Geometry: final body of the model. Coordinates: model frame, mm. A direction names the side the tool comes from. Coordinates: 2 decimals unless noted, no trailing zeros. Write each loop counter-clockwise with the first axis right and the second up, starting at its lowest first coordinate (ties: lowest second). Pieces come first, ordered by that corner, then holes. Notation, with made-up numbers: (6.5, 47) -> (23.5, 47) arc R17 ccw to (23.5, 78) -> close; hole circle Ø5 at (20, 77.25). An arc over 180 degrees is marked (long way). One line per item, written item: value.
```python
from build123d import *

# Parameters (mm, degrees)
SKETCH_1_R          = 27.5
EXTRUDE_1_DEPTH     = 4
SKETCH_2_R          = 25.4
EXTRUDE_2_DEPTH     = 3.175
SKETCH_3_R          = 1.6
CUT_EXTRUDE_1_DEPTH = 40.547194907
SKETCH_4_R          = 36
SKETCH_4_R_2        = 1.6
EXTRUDE_3_DEPTH     = 2


with BuildPart() as part:
    # ｽｹｯﾁ1 → ﾎﾞｽ - 押し出し1 (new body)
    with BuildSketch(Plane.XY):
        Circle(SKETCH_1_R)
    extrude(amount=EXTRUDE_1_DEPTH)

    # ｽｹｯﾁ2 → ﾎﾞｽ - 押し出し2 (add)
    with BuildSketch(Plane(origin=(0, 0, 0), x_dir=(-1, 0, 0), z_dir=(0, 0, -1))):
        Circle(SKETCH_2_R)
    extrude(amount=EXTRUDE_2_DEPTH)

    # ｽｹｯﾁ3 → ｶｯﾄ - 押し出し1 (cut, through all)
    with BuildSketch(Plane(origin=(0, 0, -3.175), x_dir=(-1, 0, 0), z_dir=(0, 0, -1))):
        with Locations((0, 22.5)):
            Circle(SKETCH_3_R)
        with Locations((22.5, 0)):
            Circle(SKETCH_3_R)
        with Locations((0, -22.5)):
            Circle(SKETCH_3_R)
        with Locations((-22.5, 0)):
            Circle(SKETCH_3_R)
    extrude(amount=-CUT_EXTRUDE_1_DEPTH, mode=Mode.SUBTRACT)

    # ｽｹｯﾁ4 → ﾎﾞｽ - 押し出し3 (add)
    with BuildSketch(Plane.XY.offset(4)):
        Circle(SKETCH_4_R)
        with Locations(Location((0, 22.5, 0), (0, 0, 180))):
            Circle(SKETCH_4_R_2, mode=Mode.SUBTRACT)
        with Locations(Location((-22.5, 0, 0), (0, 0, 180))):
            Circle(SKETCH_4_R_2, mode=Mode.SUBTRACT)
        with Locations(Location((0, -22.5, 0), (0, 0, 180))):
            Circle(SKETCH_4_R_2, mode=Mode.SUBTRACT)
        with Locations(Location((22.5, 0, 0), (0, 0, 180))):
            Circle(SKETCH_4_R_2, mode=Mode.SUBTRACT)
    extrude(amount=EXTRUDE_3_DEPTH)


solid = part.part
```
(1) Section A-A (y = 0). Return the cut outline in (x, z) (3 decimals), then the cut area to 3 significant figures.
Responses:
outline: (-36, 4) -> (-27.5, 4) -> (-27.5, 0) -> (-25.4, 0) -> (-25.4, -3.175) -> (-24.1, -3.175) -> (-24.1, 6) -> (-36, 6) -> close; (-20.9, -3.175) -> (20.9, -3.175) -> (20.9, 6) -> (-20.9, 6) -> close; (24.1, -3.175) -> (25.4, -3.175) -> (25.4, 0) -> (27.5, 0) -> (27.5, 4) -> (36, 4) -> (36, 6) -> (24.1, 6) -> close
area: 467 mm2
(2) Section B-B (z = 2.25). Return the cut outline in (x, y).
Responses:
outline: circle Ø55 at (0, 0); hole circle Ø3.2 at (-22.5, 0); hole circle Ø3.2 at (0, -22.5); hole circle Ø3.2 at (0, 22.5); hole circle Ø3.2 at (22.5, 0)
(3) Line query: line 1 (Y direction, x = 0, z = 3); line 2 (Y direction, x = -22.5, z = 0.5); line 3 (Z direction, x = 25.5, y = 5). Output: solid intervals per line, ascending. Write a range as [from, to].
Responses:
line 1: y = [-27.5, -24.1], [-20.9, 20.9], [24.1, 27.5]
line 2: y = [-15.81, -1.6], [1.6, 15.81]
line 3: z = [0, 6]
(4) First-contact query: pin 1 (4 mm diameter, centred on x = 10, z = 5, fed in from -Y); pin 2 (4 mm diameter, centred on y = 25.5, z = 4, fed in from +X); pin 3 (2.5 mm diameter, centred on x = -22.5, y = 0, fed in from +Z); pin 4 (1 mm diameter, centred on x = 20, z = -1.5, fed in from +Y). Flat tips, straight axial feed; report the tip coordinate or a pass-through.
Responses:
pin 1: stops at y = -35.1
pin 2: stops at x = 27.27
pin 3: passes through
pin 4: stops at y = 16.28
(5) Section C-C (x = -22.5). Return the cut outline in (y, z) (1 decimal), then the cut area to 3 significant figures.
Responses:
outline: (-28.1, 4) -> (-15.8, 4) -> (-15.8, 0) -> (-11.8, 0) -> (-11.8, -3.2) -> (-1.6, -3.2) -> (-1.6, 6) -> (-28.1, 6) -> close; (1.6, -3.2) -> (11.8, -3.2) -> (11.8, 0) -> (15.8, 0) -> (15.8, 4) -> (28.1, 4) -> (28.1, 6) -> (1.6, 6) -> close
area: 284 mm2
(6) Reachability of faces 1 (the flat face through (0, 0, -3.175)), 2 (the cylindrical face through (-5.961, -26.846, 1.972)) from +Z, -Z, +X, -X, +Y, -Y: full face, straight path, thin tool, end or side. Return the list, or none.
Responses:
face 1: -Z, +X, -X, +Y, -Y
face 2: -Z
(7) Pull-direction query (Y, two-part tool) for faces 3 (the cylindrical face through (0.208, -24.086, 1.348)), 4 (the flat face through (-1, 1, 6)), 5 (the cylindrical face through (-4.686, 35.694, 4.986)), 6 (the cylindrical face through (0.208, 20.914, 1.348)); classes: released by +Y, released by -Y, zero draft, split by the parting line, or undercut.
Responses:
face 3: undercut
face 4: zero draft
face 5: split by the parting line
face 6: undercut
